Check sheet for the modelled part. Datum: model origin and axes. Units: mm. A direction names the side the tool comes from. Round coordinates to 2 decimals unless told otherwise and drop trailing zeros. Write each loop counter-clockwise with the first axis right and the second up, starting at its lowest first coordinate (ties: lowest second). Pieces come first, ordered by that corner, then holes. Notation, with made-up numbers: (-31.5, -29.75) -> (-10.5, -29.75) arc R4 ccw to (-10.5, -24.75) -> close; hole circle Ø4 at (44.25, 77.5). An arc over 180 degrees is marked (long way). One line per item, written item: value.
from build123d import *

# Parameters (mm, degrees)
MODEL_R             = 1.300000002
MODEL_R_2           = 1.299950005
MODEL_R_3           = 1.299950001
MODEL_W             = 11.8
MODEL_H             = 23
BOSS_EXTRUDE1_DEPTH = 3


with BuildPart() as part:
    # Model → Boss-Extrude1 (new body)
    with BuildSketch(Plane.XY):
        with BuildLine():
            Line((33.3225, 20.129700001), (33.3225, 64.129600001))
            ThreePointArc((33.3225, 64.129600001), (34.136296645, 66.222490163), (36.19171658, 67.126759536))
            Line((36.19171658, 67.126759536), (80.3225, 67.129600001))
            ThreePointArc((80.3225, 67.129600001), (82.4438375, 66.250937501), (83.3225, 64.129600001))
            Line((83.3225, 64.129600001), (83.3225, 20.129700001))
            ThreePointArc((83.3225, 20.129700001), (82.443835355, 18.008335356), (80.3225, 17.129600001))
            Line((80.3225, 17.129600001), (36.3225, 17.129600001))
            ThreePointArc((36.3225, 17.129600001), (34.201114643, 18.008285356), (33.3225, 20.129700001))
        make_face()
        with Locations((36.322500002, 64.129699999)):
            Circle(MODEL_R, mode=Mode.SUBTRACT)
        with Locations((80.322500002, 64.129699999)):
            Circle(MODEL_R, mode=Mode.SUBTRACT)
        with Locations((67.322549996, 42.129649997)):
            Circle(MODEL_R_2, mode=Mode.SUBTRACT)
        with Locations((49.32245, 42.129650001)):
            Circle(MODEL_R_3, mode=Mode.SUBTRACT)
        with Locations((36.322549996, 20.129649997)):
            Circle(MODEL_R_2, mode=Mode.SUBTRACT)
        with Locations((80.322549996, 20.129649997)):
            Circle(MODEL_R_2, mode=Mode.SUBTRACT)
        with Locations((58.3225, 42.129600001)):
            Rectangle(MODEL_W, MODEL_H, mode=Mode.SUBTRACT)
    extrude(amount=BOSS_EXTRUDE1_DEPTH)


solid = part.part
Item 1: Sectioned sample at C-C on z = 2.1. Enter the section's corners in (x, y), and give its area (3 significant figures).
Answer:
outline: (33.32, 20.13) arc R3 ccw to (36.32, 17.13) -> (80.32, 17.13) arc R3 ccw to (83.32, 20.13) -> (83.32, 64.13) arc R3 ccw to (80.32, 67.13) -> (36.19, 67.13) arc R2.93 ccw to (33.32, 64.13) -> close; hole circle Ø2.6 at (36.32, 20.13); hole circle Ø2.6 at (36.32, 64.13); hole circle Ø2.6 at (49.32, 42.13); hole (52.42, 30.63) -> (64.22, 30.63) -> (64.22, 53.63) -> (52.42, 53.63) -> close; hole circle Ø2.6 at (67.32, 42.13); hole circle Ø2.6 at (80.32, 20.13); hole circle Ø2.6 at (80.32, 64.13)
area: 2,190 mm^2
Item 2: Mould release check, pull along Y, two halves, no side actions. Record for faces 3 (the flat face through (59, 17.13, 1)), 4 (the cylindrical face through (48.364, 43.008, 1.479)), 5 (the cylindrical face through (82.42, 66.274, 1.479)): pulls with the +Y half, pulls with the -Y half, needs draft (parallel to the pull), parting line crosses it, or undercut.
Answer:
face 3: pulls with the -Y half
face 4: undercut
face 5: pulls with the +Y half
Item 3: Thickness scan on line 1 (X direction, y = 42, z = 1.75); line 2 (Y direction, x = 60.5, z = 0.3); line 3 (X direction, y = 49, z = 2). Record the ranges inside material, lowest first.
Answer:
line 1: x = 33.32 to 48.03, 50.62 to 52.42, 64.22 to 66.03, 68.62 to 83.32
line 2: y = 17.13 to 30.63, 53.63 to 67.13
line 3: x = 33.32 to 52.42, 64.22 to 83.32
Item 4: Sectioned sample at B-B on x = 60. Enter the section's corners in (y, z).
Answer:
outline: (17.13, 0) -> (30.63, 0) -> (30.63, 3) -> (17.13, 3) -> close; (53.63, 0) -> (67.13, 0) -> (67.13, 3) -> (53.63, 3) -> close
Item 5: Tool access check on faces 1 (the flat face through (58, 53.63, 1)), 2 (the cylindrical face through (82.467, 18.032, 1.479)). Record the directions out of +Z, -Z, +X, -X, +Y, -Y that give a thin tool (end or side, any length) a straight path to the whole face; none if there is none.
Answer:
face 1: +Z, -Z
face 2: +Z, -Z, +X, -Y
Item 6: Sectioned sample at A-A on y = 53. Enter the section's corners in (x, z).
Answer:
outline: (33.32, 0) -> (52.42, 0) -> (52.42, 3) -> (33.32, 3) -> close; (64.22, 0) -> (83.32, 0) -> (83.32, 3) -> (64.22, 3) -> close
Item 7: Depth check by flat-ended pin: P1, Ø2.5, axis at x = 36.32, y = 64.13, coming from the +Z side. Enter the tip coordinate at first touch or a pass-through.
Answer:
P1: passes through
